from build123d import *

# Parameters (mm, degrees)
F0_W     = 200
F0_H     = 200
F1_DEPTH = 5
F2_W     = 10
F2_H     = 10
F2_W_2   = 190
F2_H_2   = 180
F3_DEPTH = 100
F5_DEPTH = 5
F6_W     = 5
F6_H     = 4.7
F7_DEPTH = 25
F6_H_2   = 4.3
F8_DEPTH = 5
F9_R     = 5


with BuildPart() as f1:
    # F0 (on Top) → F1 (new body)
    with BuildSketch(Plane.XY):
        Rectangle(F0_W, F0_H)
    extrude(amount=F1_DEPTH)

    # F2 (on face) → F3 (join)
    with BuildSketch(Plane.XY.offset(5)):
        with Locations((-95, 95)):
            Rectangle(F2_W, F2_H)
        with Locations((5, 95)):
            Rectangle(F2_W_2, F2_H)
        with Locations((-95, 0)):
            Rectangle(F2_W, F2_H_2)
        with Locations((-95, -95)):
            Rectangle(F2_W, F2_H)
        with Locations((5, -95)):
            Rectangle(F2_W_2, F2_H)
    extrude(amount=F3_DEPTH)

    # F4 (on face) → F5 (cut)
    with BuildSketch(Plane.XY.offset(105)):
        Polygon((100, 90), (100, 95), (-95, 95), (-95, -95), (100, -95), (100, -90), (-90, -90), (-90, 90), align=None)
    extrude(amount=-F5_DEPTH, mode=Mode.SUBTRACT)

    # F6 (on face) → F7 (cut)
    with BuildSketch(Plane.XY.offset(5)):
        with Locations((97.5, -83.35)):
            Rectangle(F6_W, F6_H)
        with Locations((97.5, -74.35)):
            Rectangle(F6_W, F6_H)
        with Locations((97.5, -65.35)):
            Rectangle(F6_W, F6_H)
        with Locations((97.5, -56.35)):
            Rectangle(F6_W, F6_H)
        with Locations((97.5, -47.35)):
            Rectangle(F6_W, F6_H)
        with Locations((97.5, -38.35)):
            Rectangle(F6_W, F6_H)
        with Locations((97.5, -29.35)):
            Rectangle(F6_W, F6_H)
        with Locations((97.5, -20.35)):
            Rectangle(F6_W, F6_H)
        with Locations((97.5, -11.35)):
            Rectangle(F6_W, F6_H)
        with Locations((97.5, -2.35)):
            Rectangle(F6_W, F6_H)
        with Locations((97.5, 6.65)):
            Rectangle(F6_W, F6_H)
        with Locations((97.5, 15.65)):
            Rectangle(F6_W, F6_H)
        with Locations((97.5, 24.65)):
            Rectangle(F6_W, F6_H)
        with Locations((97.5, 33.65)):
            Rectangle(F6_W, F6_H)
        with Locations((97.5, 42.65)):
            Rectangle(F6_W, F6_H)
        with Locations((97.5, 51.65)):
            Rectangle(F6_W, F6_H)
        with Locations((97.5, 60.65)):
            Rectangle(F6_W, F6_H)
        with Locations((97.5, 69.65)):
            Rectangle(F6_W, F6_H)
        with Locations((97.5, 78.65)):
            Rectangle(F6_W, F6_H)
        with Locations((97.5, 87.65)):
            Rectangle(F6_W, F6_H)
    extrude(amount=-F7_DEPTH, mode=Mode.SUBTRACT)

    # F6 (on face) → F8 (join)
    with BuildSketch(Plane.XY.offset(5)):
        with Locations((102.5, -87.85)):
            Rectangle(F6_W, F6_H_2)
        with Locations((102.5, -78.85)):
            Rectangle(F6_W, F6_H_2)
        with Locations((102.5, -69.85)):
            Rectangle(F6_W, F6_H_2)
        with Locations((102.5, -60.85)):
            Rectangle(F6_W, F6_H_2)
        with Locations((102.5, -51.85)):
            Rectangle(F6_W, F6_H_2)
        with Locations((102.5, -42.85)):
            Rectangle(F6_W, F6_H_2)
        with Locations((102.5, -33.85)):
            Rectangle(F6_W, F6_H_2)
        with Locations((102.5, -24.85)):
            Rectangle(F6_W, F6_H_2)
        with Locations((102.5, -15.85)):
            Rectangle(F6_W, F6_H_2)
        with Locations((102.5, -6.85)):
            Rectangle(F6_W, F6_H_2)
        with Locations((102.5, 2.15)):
            Rectangle(F6_W, F6_H_2)
        with Locations((102.5, 11.15)):
            Rectangle(F6_W, F6_H_2)
        with Locations((102.5, 20.15)):
            Rectangle(F6_W, F6_H_2)
        with Locations((102.5, 29.15)):
            Rectangle(F6_W, F6_H_2)
        with Locations((102.5, 38.15)):
            Rectangle(F6_W, F6_H_2)
        with Locations((102.5, 47.15)):
            Rectangle(F6_W, F6_H_2)
        with Locations((102.5, 56.15)):
            Rectangle(F6_W, F6_H_2)
        with Locations((102.5, 65.15)):
            Rectangle(F6_W, F6_H_2)
        with Locations((102.5, 74.15)):
            Rectangle(F6_W, F6_H_2)
        with Locations((102.5, 83.15)):
            Rectangle(F6_W, F6_H_2)
    extrude(amount=-F8_DEPTH)

    # F9
    f9_edges = [f1.edges().sort_by_distance(p)[0] for p in [
        (-100, -100, 52.5),
        (-100, 100, 52.5),
    ]]
    fillet(f9_edges, radius=F9_R)


solid = f1.part
Could you check a few things on this model? Use its own coordinates, in mm. A direction names the side the tool comes from. Give positions to 0.01 mm unless a question says otherwise; leave off trailing zeros. Loops run counter-clockwise (first coordinate to the right, second up) from the corner with the lowest first, then second, coordinate; pieces in that order, holes last. Notation, with made-up numbers: (56.25, 52) -> (111.25, 52) arc R20 ccw to (111.25, 84) -> close; hole circle Ø3 at (19, -38). An arc over 180 degrees is marked (long way). Answer as CSV lines item,"result". Start each with the question number.
(1) I'm going to push flat-ended pins straight in: pin 1 Ø4 at (x, z) = (102.5, 2.5) entering from +Y; pin 2 Ø5 at (y, z) = (96.5, 47) entering from +X; pin 3 Ø4 at (x, y) = (-8.5, 36.5) entering from +Z. Where does each tip first touch, or does it pass through?
(2) If we section it at A-A on x = 58: Write out the boundary of the cut face in (y, z), then the cut area to 3 significant figures.
(3) We'd pull the mould along Y, two halves only. Please class faces 1 (the flat face through (100, -40.7, 3)), 2 (the flat face through (100, -95, 52)): released by +Y, released by -Y, zero draft, split by the parting line, or undercut.
(4) If we section it at B-B on z = 32: Write out the boundary of the cut face in (x, y).
(5) I need wall thicknesses on probe 1 along Y at (x, z) = (0.5, 11); probe 2 along X at (y, z) = (6, 58.5); probe 3 along Z at (x, y) = (25.5, 10). Which ranges of each line are inside material? Lowest first, please.
(6) Which directions (+Z, -Z, +X, -X, +Y, -Y) give clear straight access to the entire face, cutting with the end or side of a thin tool? Please do faces 3 (the flat face through (100, -45, 3)), 4 (the flat face through (-90, -1, 52)).
Computed:
1,pin 1,"stops at y = 85.3"
1,pin 2,"stops at x = 100"
1,pin 3,"stops at z = 5"
2,outline,"(-100, 0) -> (100, 0) -> (100, 105) -> (95, 105) -> (95, 100) -> (90, 100) -> (90, 5) -> (-90, 5) -> (-90, 100) -> (-95, 100) -> (-95, 105) -> (-100, 105) -> close"
2,area,"2,950 mm2"
3,face 1,"undercut"
3,face 2,"zero draft"
4,outline,"(-100, -95) arc R5 ccw to (-95, -100) -> (100, -100) -> (100, -90) -> (-90, -90) -> (-90, 90) -> (100, 90) -> (100, 100) -> (-95, 100) arc R5 ccw to (-100, 95) -> close"
5,probe 1,"y = -100 to -90, 90 to 100"
5,probe 2,"x = -100 to -90"
5,probe 3,"z = 0 to 5"
6,face 3,"+Z, -Z, +X"
6,face 4,"+Z, +X"
